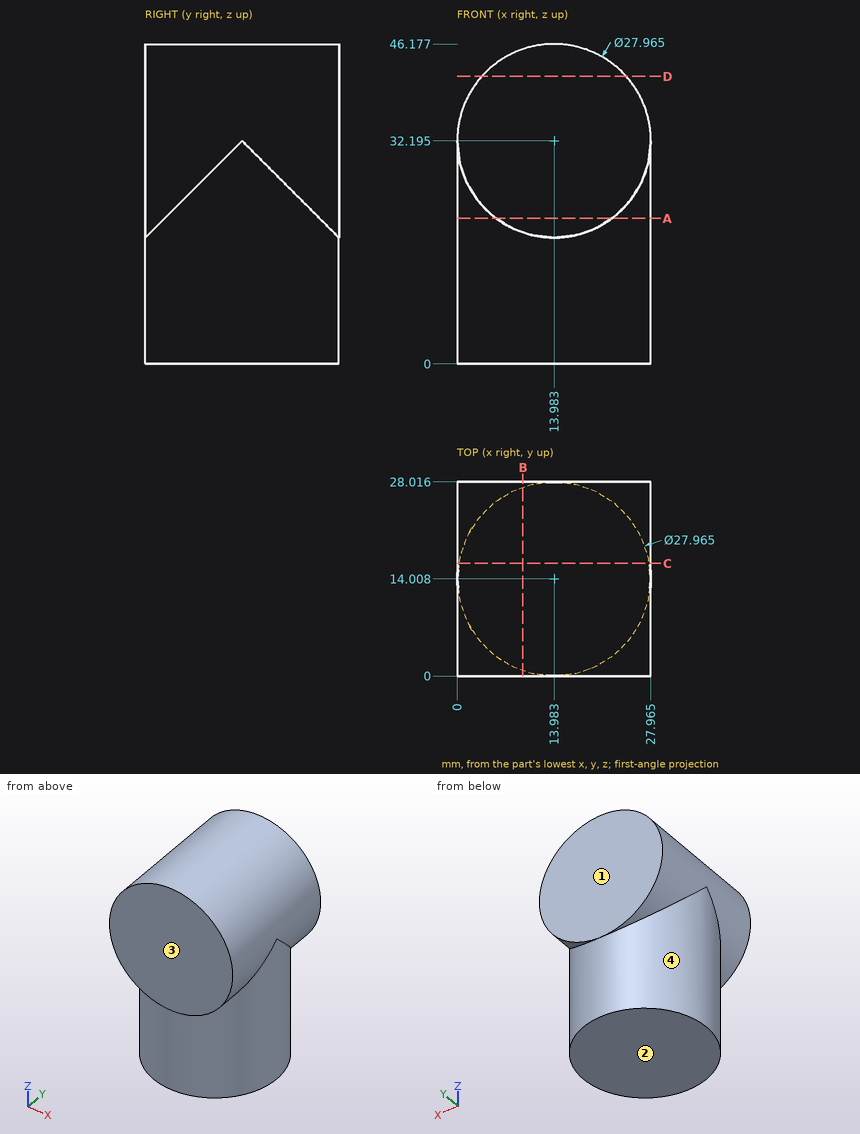
Can you work these out from the drawing? Everything is in mm from the part's minimum corner. Round coordinates to 2 decimals unless told otherwise and drop trailing zeros. Order: outer loops, then holes, each group sorted by start corner. A loop starts at its lowest first (then second) coordinate and runs counter-clockwise, first axis right, second up. Notation, with made-up numbers: (55.25, 15) -> (64.25, 15) arc R15 ccw to (64.25, 42) -> close; hole circle Ø7 at (18.25, 15.25). An arc over 180 degrees is marked (long way). Use CSV: the item, a comma, the result in double quotes.
1. I need wall thicknesses on line 1 along X through (y, z) = (25, 32) (1 decimal); line 2 along X through (y, z) = (20, 38.5); line 3 along Z through (x, y) = (22, 7.75). Which ranges of each line are inside material? Lowest first, please.
Recorded:
line 1,"x = 0 to 28"
line 2,"x = 1.5 to 26.46"
line 3,"z = 0 to 43.65"
2. Thinking about a two-plate mould opening in Y: for the marked faces 1, 2, 3 and 4, which applies, pulls with the +Y half, pulls with the -Y half, needs draft (parallel to the pull), parting line crosses it, or undercut?
Recorded:
face 1,"pulls with the +Y half"
face 2,"needs draft"
face 3,"pulls with the -Y half"
face 4,"parting line crosses it"
3. I want a section at C-C on y = 16.25. List the corners of the cut face in (x, z) for me (1 decimal), and give its area (3 significant figures).
Recorded:
outline,"(0.2, 0) -> (27.8, 0) -> (27.8, 30) arc R14 ccw (long way) to (0.2, 30) -> close"
area,"1,200 mm2"
4. I want a section at B-B on x = 9.5. List the corners of the cut face in (y, z) for me, and give its area (3 significant figures).
Recorded:
outline,"(0, 18.95) -> (0.76, 18.95) -> (0.76, 0) -> (27.25, 0) -> (27.25, 18.95) -> (28.02, 18.95) -> (28.02, 45.44) -> (0, 45.44) -> close"
area,"1,240 mm2"
5. I want a section at A-A on z = 21. List the corners of the cut face in (x, y) for me (1 decimal).
Recorded:
outline,"(5.6, 0) -> (22.4, 0) -> (22.4, 2.8) arc R14 ccw to (22.4, 25.2) -> (22.4, 28) -> (5.6, 28) -> (5.6, 25.2) arc R14 ccw to (5.6, 2.8) -> close"
6. I want a section at D-D on z = 41.5. List the corners of the cut face in (x, y) for me, and give its area (3 significant figures).
Recorded:
outline,"(3.55, 0) -> (24.42, 0) -> (24.42, 28.02) -> (3.55, 28.02) -> close"
area,"585 mm2"
7. I'm going to push flat-ended pins straight in: P1, Ø2, axis at y = 5.5, z = 16, coming from the +X side; P2, Ø10, axis at y = 5, z = 10, coming from the -X side; P3, Ø1, axis at y = 6, z = 18.5, coming from the -X side; P4, Ø10, axis at x = 13.5, y = 14.5, coming from the -Z side. Where does each tip first touch, or does it pass through?
Recorded:
P1,"stops at x = 25.78"
P2,"stops at x = 0.59"
P3,"stops at x = 2.19"
P4,"stops at z = 0"
